from build123d import *

# Parameters (mm, degrees)
BOSS_EXTRUDE1_DEPTH = 3
SKETCH4_W           = 144.4
SKETCH4_H           = 3
CUT_EXTRUDE1_DEPTH  = 4
SKETCH5_W           = 20.628571
SKETCH5_H           = 3
BOSS_EXTRUDE2_DEPTH = 3


with BuildPart() as part:
    # Sketch2 → Boss-Extrude1 (new body)
    with BuildSketch(Plane(origin=(0, 0, 0), x_dir=(1, 0, 0), z_dir=(0, 1, 0))):
        Polygon((-69.2, -68.5), (-41.52, -68.5), (-41.52, -71.5), (-13.84, -71.5), (-13.84, -68.5), (13.84, -68.5), (13.84, -71.5), (41.52, -71.5), (41.52, -68.5), (69.2, -68.5), (69.2, -45.653333333), (72.2, -45.653333333), (72.2, -22.823333333), (69.2, -22.823333333), (69.2, 0.006666667), (72.2, 0.006666667), (72.2, 22.836666667), (69.2, 22.836666667), (69.2, 45.666666667), (72.2, 45.666666667), (72.2, 68.5), (-72.2, 68.5), (-72.2, 45.666666667), (-69.2, 45.666666667), (-69.2, 22.836666667), (-72.2, 22.836666667), (-72.2, 0.006666667), (-69.2, 0.006666667), (-69.2, -22.823333333), (-72.2, -22.823333333), (-72.2, -45.653333333), (-69.2, -45.653333333), align=None)
    extrude(amount=BOSS_EXTRUDE1_DEPTH)

    # Sketch4 → Cut-Extrude1 (cut, through all)
    with BuildSketch(Plane.XZ):
        with Locations((0, -67)):
            Rectangle(SKETCH4_W, SKETCH4_H)
    extrude(amount=-CUT_EXTRUDE1_DEPTH, mode=Mode.SUBTRACT)

    # Sketch5 → Boss-Extrude2 (add)
    with BuildSketch(Plane.XZ):
        with Locations((-41.257143071, -67)):
            Rectangle(SKETCH5_W, SKETCH5_H)
        with Locations((-1.071e-06, -67)):
            Rectangle(SKETCH5_W, SKETCH5_H)
        with Locations((41.257140929, -67)):
            Rectangle(SKETCH5_W, SKETCH5_H)
    extrude(amount=-BOSS_EXTRUDE2_DEPTH)


solid = part.part
The listing builds one solid part. Answer for the finished solid, in the listing's coordinates (mm). Round coordinates to 2 decimals unless told otherwise and drop trailing zeros. Order: outer loops, then holes, each group sorted by start corner. A loop starts at its lowest first (then second) coordinate and runs counter-clockwise, first axis right, second up. Notation, with made-up numbers: (19, 20) - (55, 20) arc R14 ccw to (55, 40) - close; hole circle Ø3 at (69, 44). An arc over 180 degrees is marked (long way). Write item = value, one per line. Start each with the question number.
1) Section A-A, the plane x = 12 is taken. Write down the section's boundary in (y, z), plus the area to 3 significant figures.
2) Section B-B, the plane z = -44 is taken. Write down the section's boundary in (x, y).
3) Given pin 1 (1.5 mm diameter, centred on y = 1, z = -38, fed in from -X); pin 2 (1.5 mm diameter, centred on y = 2, z = 70, fed in from -X); pin 3 (0.9 mm diameter, centred on x = 53, y = 1.5, fed in from +Z), each flat-ended and moving along its own axis, determine where each tip first touches the part or whether it passes through.
4) Straight lines are drawn through the part: L1, parallel to Z at x = 55, y = 0.9; L2, parallel to Z at x = 46.5, y = 2.75; L3, parallel to X at y = 1.7, z = 62.5. For each, find the intervals that lie inside material, in ascending order.
Results list:
q1.outline = (0, -65.5) - (3, -65.5) - (3, 68.5) - (0, 68.5) - close
q1.area = 402 mm^2
q2.outline = (-69.2, 0) - (69.2, 0) - (69.2, 3) - (-69.2, 3) - close
q3.pin_1 = -69.2
q3.pin_2 = -41.52
q3.pin_3 = 68.5
q4.L1 = -65.5 to 68.5
q4.L2 = -68.5 to 68.5
q4.L3 = -69.2 to 69.2
